```python
from build123d import *

# Parameters (mm, degrees)
BOSS_EXTRU_1_DEPTH      = 93
ESQUISSE2_R             = 1.6
ENL_V_MAT_EXTRU_1_DEPTH = 121.966784717


with BuildPart() as part:
    # Esquisse1 → Boss.-Extru.1 (new body)
    with BuildSketch(Plane.XY):
        Polygon((-20, -469.409867617), (-59.025104869, -469.409867617), (-59.025104869, -464.409867617), (0, -464.409867617), (0, -469.409867617), (-15, -469.409867617), (-15, -509.409867617), (0, -509.409867617), (0, -514.409867617), (-20, -514.409867617), align=None)
    extrude(amount=-BOSS_EXTRU_1_DEPTH)

    # Esquisse2 → Enlèv. mat.-Extru.1 (cut, through all)
    with BuildSketch(Plane(origin=(0, -464.409867617, 0), x_dir=(1, 0, 0), z_dir=(0, 1, 0))):
        with Locations(Location((-40.025104869, 90.5, 0), (0, 0, 270))):
            Circle(ESQUISSE2_R)
        with Locations(Location((-40.025104869, 2.5, 0), (0, 0, 270))):
            Circle(ESQUISSE2_R)
    extrude(amount=-ENL_V_MAT_EXTRU_1_DEPTH, mode=Mode.SUBTRACT)


solid = part.part
```
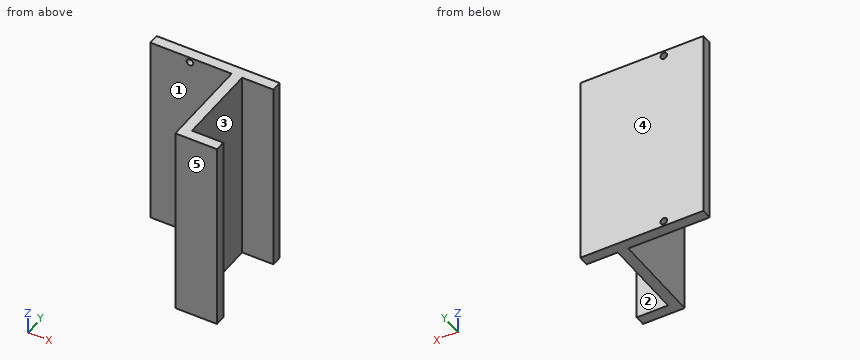
Work out the finished part from the listing and answer in its coordinate system (mm). Face numbers are marked on the shaded views. A direction names the side the tool comes from. Round coordinates to 2 decimals unless told otherwise and drop trailing zeros. Loops run counter-clockwise (first coordinate to the right, second up) from the corner with the lowest first, then second, coordinate; pieces in that order, holes last. Notation, with made-up numbers: (60.5, 49.5) -> (108.5, 49.5) arc R12 ccw to (108.5, 67.5) -> close; hole circle Ø10 at (-26, 55). An arc over 180 degrees is marked (long way). Write each question's results on one line, items separated by ' | '. Start each with the question number.
1. A tool of negligible diameter and unlimited length cuts with its end or side. For the marked faces 1 and 2, from which of +Z, -Z, +X, -X, +Y, -Y can it reach the whole face along a straight path? Write none if from no direction.
2. For a pull along Y with two mould halves and no side action, classify the marked faces 3, 4 and 5 as +Y half, -Y half, draft (parallel to the pull), parting line (faces both ways), or undercut.
3. Section D-D (y = -474.5) is taken. Determine the outline of the cut face in (x, z).
4. Section A-A (z = -90.5) is taken. Determine the outline of the cut face in (x, y).
5. Section B-B (x = -8) is taken. Determine the outline of the cut face in (y, z).
6. Given pin 1 Ø13.5 at (y, z) = (-482.5, -25) entering from -X; pin 2 Ø20 at (y, z) = (-484.5, -25.5) entering from +X; pin 3 Ø5 at (x, z) = (-40.03, -2.5) entering from -Y; pin 4 Ø3 at (x, z) = (-40.03, -90.5) entering from -Y, each flat-ended and moving along its own axis, determine where each tip first touches the part or whether it passes through.
7. Section C-C (z = -72) is taken. Determine the outline of the cut face in (x, y).
8. Find the intervals of material crossed by probe 1 along Y at (x, z) = (-6, -63.5); probe 2 along X at (y, z) = (-467.4, -90.5); probe 3 along Y at (x, z) = (-34, -89), in increasing order. Write a range as from..to.
Evaluation:
1) face 1: +Z, -Z, -X, -Y | face 2: +Z, -Z, +X
2) face 3: undercut | face 4: +Y half | face 5: -Y half
3) outline: (-20, -93) -> (-15, -93) -> (-15, 0) -> (-20, 0) -> close
4) outline: (-59.03, -469.41) -> (-41.63, -469.41) -> (-41.63, -464.41) -> (-59.03, -464.41) -> close; (-38.43, -469.41) -> (-20, -469.41) -> (-20, -514.41) -> (0, -514.41) -> (0, -509.41) -> (-15, -509.41) -> (-15, -469.41) -> (0, -469.41) -> (0, -464.41) -> (-38.43, -464.41) -> close
5) outline: (-514.41, -93) -> (-509.41, -93) -> (-509.41, 0) -> (-514.41, 0) -> close; (-469.41, -93) -> (-464.41, -93) -> (-464.41, 0) -> (-469.41, 0) -> close
6) pin 1: stops at x = -20 | pin 2: stops at x = -15 | pin 3: stops at y = -469.41 | pin 4: passes through
7) outline: (-59.03, -469.41) -> (-20, -469.41) -> (-20, -514.41) -> (0, -514.41) -> (0, -509.41) -> (-15, -509.41) -> (-15, -469.41) -> (0, -469.41) -> (0, -464.41) -> (-59.03, -464.41) -> close
8) probe 1: y = -514.41..-509.41, -469.41..-464.41 | probe 2: x = -59.03..-41.63, -38.43..0 | probe 3: y = -469.41..-464.41
